```python
from build123d import *

# Parameters (mm, degrees)
CROQUIS1_R                   = 55
DISCO_DEPTH                  = 5
CORTAR_EXTRUIR1_DEPTH        = 10
SALIENTE_EXTRUIR1_DEPTH      = 10
SALIENTE_EXTRUIR1_DEPTH_BACK = 5
CROQUIS7_R                   = 60
CROQUIS7_R_2                 = 55
CROQUIS7_R_3                 = 53
SALIENTE_EXTRUIR6_DEPTH      = 5


with BuildPart() as part:
    # Croquis1 → Disco (new body)
    with BuildSketch(Plane.XY):
        Circle(CROQUIS1_R)
    extrude(amount=DISCO_DEPTH)

    # Croquis6 → Cortar-Extruir1 (cut)
    with BuildSketch(Plane.XY.offset(5)):
        with BuildLine():
            Line((-5.25, 0), (-5.25, -30))
            ThreePointArc((-5.25, -30), (0, -35.25), (5.25, -30))
            Line((5.25, -30), (5.25, 0))
            ThreePointArc((5.25, 0), (0, 5.25), (-5.25, 0))
        make_face()
        with BuildLine():
            Line((2.625, 4.54663337), (-23.355762114, 19.54663337))
            ThreePointArc((-23.355762114, 19.54663337), (-30.527395483, 17.625), (-28.605762114, 10.45336663))
            Line((-28.605762114, 10.45336663), (-2.625, -4.54663337))
            ThreePointArc((-2.625, -4.54663337), (4.54663337, -2.625), (2.625, 4.54663337))
        make_face()
        with BuildLine():
            Line((2.625, -4.54663337), (28.605762114, 10.45336663))
            ThreePointArc((28.605762114, 10.45336663), (30.527395483, 17.625), (23.355762114, 19.54663337))
            Line((23.355762114, 19.54663337), (-2.625, 4.54663337))
            ThreePointArc((-2.625, 4.54663337), (-4.54663337, -2.625), (2.625, -4.54663337))
        make_face()
    extrude(amount=-CORTAR_EXTRUIR1_DEPTH, mode=Mode.SUBTRACT)

    # Croquis7 → Saliente-Extruir1 (add, two sides: drawn at the far end of the back side and taken through both)
    # profile 1 of 2: a face of its own
    with BuildSketch(Plane.XY.offset(5).offset(-SALIENTE_EXTRUIR1_DEPTH_BACK)):
        Circle(CROQUIS7_R)
        Circle(CROQUIS7_R_2, mode=Mode.SUBTRACT)
    # profile 2 of 2: a face of its own
    with BuildSketch(Plane.XY.offset(5).offset(-SALIENTE_EXTRUIR1_DEPTH_BACK)):
        Circle(CROQUIS7_R_2)
        Circle(CROQUIS7_R_3, mode=Mode.SUBTRACT)
    extrude(amount=SALIENTE_EXTRUIR1_DEPTH + SALIENTE_EXTRUIR1_DEPTH_BACK)

    # Croquis8 → Saliente-Extruir6 (add)
    with BuildSketch(Plane.XY.offset(5)):
        Polygon((-8.714101615, -5.031088913), (0, 10.062177826), (8.714101615, -5.031088913), align=None)
    extrude(amount=-SALIENTE_EXTRUIR6_DEPTH)


solid = part.part
```
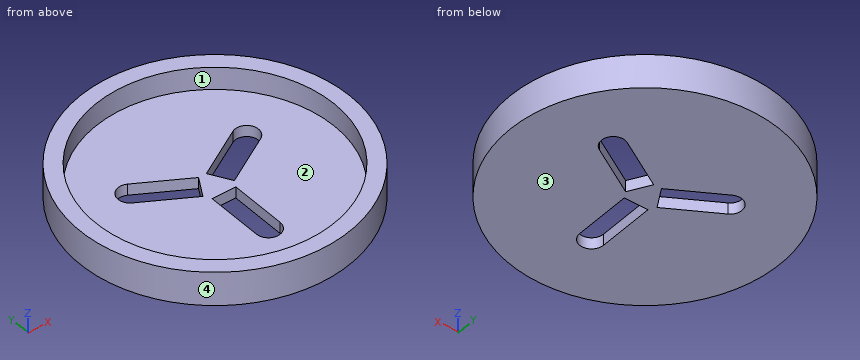
Source: CAD feature listing. Evaluate the final solid. Frame: model axes, mm. Face numbers are marked on the shaded views. Coordinates: 2 decimals unless noted, no trailing zeros. Loops run counter-clockwise (first coordinate to the right, second up) from the corner with the lowest first, then second, coordinate; pieces in that order, holes last. Notation, with made-up numbers: (39.5, -30.5) -> (50.5, -30.5) arc R25 cw to (50.5, 3.5) -> close; hole circle Ø2 at (29.25, 78). An arc over 180 degrees is marked (long way). One line per item, written item: value. Start each with the question number.
Q1. Mould query, pull axis X, two halves, no side actions, for the marked faces 1, 2, 3 and 4. Classes: pulls with the +X half, pulls with the -X half, needs draft (parallel to the pull), parting line crosses it, or undercut.
Q2. Section query A-A, the plane x = 0. Return the cut outline in (y, z).
Q3. Section query C-C, the plane z = 3.5. Return the cut outline in (x, y), and give its area (3 significant figures).
Q4. Section query D-D, the plane x = 40.5. Return the cut outline in (y, z), and give its area (3 significant figures).
Q5. Contact query for flat-ended pins moving along their axis: P1, Ø2, axis at x = -21, z = 7.5, coming from the +Y side; P2, Ø1.5, axis at y = -15, z = 5.5, coming from the +X side; P3, Ø1, axis at x = -37.5, z = 3.5, coming from the +Y side. Output: stop coordinate, or through.
Q6. Section query B-B, the plane y = 0. Return the cut outline in (x, z).
Q7. Line query: line 1 along Y through (x, z) = (0, 11.75); line 2 along X through (y, z) = (19.5, 1) (3 decimals); line 3 along Z through (x, y) = (43, -24). Output: solid intervals per line, ascending.
Results:
1. face 1: undercut
1. face 2: undercut
1. face 3: needs draft
1. face 4: parting line crosses it
2. outline: (-60, 0) -> (-35.25, 0) -> (-35.25, 5) -> (-53, 5) -> (-53, 15) -> (-60, 15) -> close; (-5.03, 0) -> (60, 0) -> (60, 15) -> (53, 15) -> (53, 5) -> (-5.03, 5) -> close
3. outline: circle Ø120 at (0, 0); hole (-28.61, 10.45) -> (-6.98, -2.03) -> (-1.73, 7.06) -> (-23.36, 19.55) arc R5.25 ccw to start; hole (-5.25, -30) arc R5.25 ccw to (5.25, -30) -> (5.25, -5.03) -> (-5.25, -5.03) -> close; hole (1.73, 7.06) -> (6.98, -2.03) -> (28.61, 10.45) arc R5.25 ccw to (23.36, 19.55) -> close
3. area: 10,400 mm^2
4. outline: (-44.27, 0) -> (44.27, 0) -> (44.27, 15) -> (34.19, 15) -> (34.19, 5) -> (-34.19, 5) -> (-34.19, 15) -> (-44.27, 15) -> close
4. area: 644 mm^2
5. P1: y = 56.57
5. P2: x = 58.28
5. P3: y = 47.23
6. outline: (-60, 0) -> (-10.5, 0) -> (-10.5, 5) -> (-53, 5) -> (-53, 15) -> (-60, 15) -> close; (-5.81, 0) -> (5.81, 0) -> (5.81, 5) -> (-5.81, 5) -> close; (10.5, 0) -> (60, 0) -> (60, 15) -> (53, 15) -> (53, 5) -> (10.5, 5) -> close
7. line 1: -60 to -53, 53 to 60
7. line 2: -56.743 to -28.685, -23.275 to 23.275, 28.685 to 56.743
7. line 3: 0 to 5
